from build123d import *

# Parameters (mm, degrees)
F0_R     = 17.5
F1_DEPTH = 5
F2_R     = 12.5
F3_DEPTH = 50
F4_W     = 55
F4_H     = 40
F4_W_2   = 45
F4_H_2   = 30
F5_DEPTH = 25
F6_W     = 3.4094286376
F6_H     = 1.5
F8_SIZE2 = 0.5773502692
F8_SIZE  = 1


with BuildPart() as f1:
    # F0 (on Top) → F1 (new body)
    with BuildSketch(Plane.XY):
        Circle(F0_R)
    extrude(amount=F1_DEPTH)

    # F2 (on face) → F3 (join)
    with BuildSketch(Plane.XY.offset(5)):
        Circle(F2_R)
    extrude(amount=F3_DEPTH)

    # F4 (on face) → F5 (cut)
    with BuildSketch(Plane(origin=(0, 0, 0), x_dir=(1, 0, 0), z_dir=(0, 0, -1))):
        Rectangle(F4_W, F4_H)
        Rectangle(F4_W_2, F4_H_2, mode=Mode.SUBTRACT)
    extrude(amount=-F5_DEPTH, mode=Mode.SUBTRACT)

    # F6 (on Right) → F7 (revolve, cut)
    with BuildSketch(Plane.YZ):
        with Locations((-13.4547143188, 35.75)):
            Rectangle(F6_W, F6_H)
    revolve(axis=Axis((0, 0, 30.1519706845), (0, 0, 1)), mode=Mode.SUBTRACT)

    # F8
    f8_edges = [f1.edges().sort_by_distance(p)[0] for p in [
        (-12.5, 0, 55),
    ]]
    f8_side = f1.faces().sort_by_distance((0, 0, 55))[0]
    chamfer(f8_edges, length=F8_SIZE, length2=F8_SIZE2, reference=f8_side)


solid = f1.part
Source: CAD feature listing. Evaluate the final solid. Frame: model axes, mm. A direction names the side the tool comes from. Round coordinates to 2 decimals unless told otherwise and drop trailing zeros. Loops run counter-clockwise (first coordinate to the right, second up) from the corner with the lowest first, then second, coordinate; pieces in that order, holes last. Notation, with made-up numbers: (14.5, -37) -> (54.5, -37) arc R15 cw to (54.5, -23) -> close; hole circle Ø10 at (34.25, 32). An arc over 180 degrees is marked (long way). Answer as a JSON object with one key per item and string values. Group by question number.
Q1. Mould query, pull axis Y, two halves, no side actions, for faces 4 (the cylindrical face through (11.923, 3.755, 19.79)), 5 (the flat face through (0, -15, 2)), 6 (the flat face through (0, 15, 2)), 7 (the flat face through (-5, -11, 35)). Classes: pulls with the +Y half, pulls with the -Y half, needs draft (parallel to the pull), parting line crosses it, or undercut.
Q2. Access query for faces 1 (the cylindrical face through (11.923, 3.755, 45.336)), 2 (the flat face through (-5, -11, 36.5)), 3 (the flat face through (0, 0, 0)). Directions: +Z, -Z, +X, -X, +Y, -Y. A direction counts if a zero-diameter tool reaches every point of the face in a straight line with its end or side. Return the directions, or none.
Q3. Section query B-B (y = 0). Output: boundary loops of the cut face in (x, z), plus the area to 3 significant figures.
Q4. Section query D-D (z = 4). Output: boundary loops of the cut face in (x, y), plus the area to 3 significant figures.
Q5. Section query C-C (z = 13). Output: boundary loops of the cut face in (x, y), plus the area to 3 significant figures.
Q6. Ray query, line 1 (Z direction, x = -13.5, y = 0); line 2 (Y direction, x = 3, z = 23); line 3 (Y direction, x = -10.5, z = 40). Return the intervals inside material, ascending. Write a range as from..to.
Q7. Section query A-A (x = 0). Output: boundary loops of the cut face in (y, z).
Q8. Contact query for flat-ended pins moving along their axis: P1, Ø1.5, axis at x = -9.5, z = 42.5, coming from the -Y side; P2, Ø8, axis at y = -3, z = 43.5, coming from the -X side; P3, Ø1.5, axis at y = -7.5, z = 5.5, coming from the -X side. Output: stop coordinate, or through.
Completed:
{
 "1": {"face 4": "parting line crosses it", "face 5": "pulls with the -Y half", "face 6": "pulls with the +Y half", "face 7": "needs draft"},
 "2": {"face 1": "+Z", "face 2": "none", "face 3": "-Z, +X, -X, +Y, -Y"},
 "3": {"outline": "(-17.5, 0) -> (17.5, 0) -> (17.5, 5) -> (12.5, 5) -> (12.5, 35) -> (11.75, 35) -> (11.75, 36.5) -> (12.5, 36.5) -> (12.5, 54.42) -> (11.5, 55) -> (-11.5, 55) -> (-12.5, 54.42) -> (-12.5, 36.5) -> (-11.75, 36.5) -> (-11.75, 35) -> (-12.5, 35) -> (-12.5, 5) -> (-17.5, 5) -> close", "area": "1,420 mm²"},
 "4": {"outline": "(-9.01, -15) -> (9.01, -15) arc R17.5 ccw to (9.01, 15) -> (-9.01, 15) arc R17.5 ccw to start", "area": "901 mm²"},
 "5": {"outline": "circle Ø25 at (0, 0)", "area": "491 mm²"},
 "6": {"line 1": "0..5", "line 2": "-12.13..12.13", "line 3": "-6.78..6.78"},
 "7": {"outline": "(-15, 0) -> (15, 0) -> (15, 5) -> (12.5, 5) -> (12.5, 35) -> (11.75, 35) -> (11.75, 36.5) -> (12.5, 36.5) -> (12.5, 54.42) -> (11.5, 55) -> (-11.5, 55) -> (-12.5, 54.42) -> (-12.5, 36.5) -> (-11.75, 36.5) -> (-11.75, 35) -> (-12.5, 35) -> (-12.5, 5) -> (-15, 5) -> close"},
 "8": {"P1": "y = -8.93", "P2": "x = -12.5", "P3": "x = -16.06"}
}
